```python
from build123d import *

# Parameters (mm, degrees)
BOSS_EXTRUDE1_DEPTH = 9
SHELL2_T            = -3
SKETCH3_W           = 14
SKETCH3_H           = 56
SKETCH3_W_2         = 12
SKETCH3_H_2         = 54
BOSS_EXTRUDE3_DEPTH = 6
FILLET1_R           = 5
FILLET5_R           = 5
FILLET8_R           = 0.5
FILLET9_R           = 3
FILLET10_R          = 2


with BuildPart() as part:
    # Sketch1 → Boss-Extrude1 (new, symmetric)
    with BuildSketch(Plane.YZ):
        with BuildLine():
            Line((0, 30), (-7.5, 30))
            ThreePointArc((-7.5, 30), (-15, 0), (-7.5, -30))
            Line((-7.5, -30), (0, -30))
            Line((0, -30), (0, 30))
        make_face()
    extrude(amount=BOSS_EXTRUDE1_DEPTH, both=True)

    # Shell2
    shell2_openings = [part.faces().sort_by_distance(p)[0] for p in [
        (0, 0, 0),
    ]]
    offset(amount=SHELL2_T, openings=shell2_openings, kind=Kind.INTERSECTION)

    # Sketch3 → Boss-Extrude3 (add, symmetric)
    with BuildSketch(Plane(origin=(0, 0, 0), x_dir=(-1, 0, 0), z_dir=(0, 1, 0))):
        Rectangle(SKETCH3_W, SKETCH3_H)
        Rectangle(SKETCH3_W_2, SKETCH3_H_2, mode=Mode.SUBTRACT)
    extrude(amount=BOSS_EXTRUDE3_DEPTH, both=True)

    # Fillet1
    fillet1_edges = [part.edges().sort_by_distance(p)[0] for p in [
        (0, -7.5, -30),
        (0, -7.5, 30),
    ]]
    fillet(fillet1_edges, radius=FILLET1_R)

    # Fillet5
    fillet5_edges = [part.edges().sort_by_distance(p)[0] for p in [
        (9, -2.207712898, 30),
        (-9, -2.207712898, -30),
        (9, -2.207712898, -30),
        (-9, -15, 0),
        (-9, -7.095136799, 29.221273379),
        (-9, -2.207712898, 30),
        (-9, -7.095136799, -29.221273379),
        (9, -15, 0),
        (9, -7.095136799, 29.221273379),
        (9, -7.095136799, -29.221273379),
    ]]
    fillet(fillet5_edges, radius=FILLET5_R)

    # Fillet8
    fillet8_edges = [part.edges().sort_by_distance(p)[0] for p in [
        (0, 0, 30),
        (-9, 0, 0),
        (9, 0, 0),
        (0, 0, -30),
        (7.535533906, 0, -28.535533906),
        (7.535533906, 0, 28.535533906),
        (-7.535533906, 0, -28.535533906),
        (-7.535533906, 0, 28.535533906),
    ]]
    fillet(fillet8_edges, radius=FILLET8_R)

    # Fillet9
    fillet9_edges = [part.edges().sort_by_distance(p)[0] for p in [
        (-7, 3, 28),
        (7, 3, 28),
        (7, 3, -28),
        (-7, 3, -28),
    ]]
    fillet(fillet9_edges, radius=FILLET9_R)

    # Fillet10
    fillet10_edges = [part.edges().sort_by_distance(p)[0] for p in [
        (-6, 0.164880099, 27),
        (-6, 0.164880099, -27),
        (6, 0.164880099, 27),
        (6, 0.164880099, -27),
    ]]
    fillet(fillet10_edges, radius=FILLET10_R)


solid = part.part
```
Input: part model. Units: mm. Frame: model coordinates. A direction names the side the tool comes from. Coordinates: 2 decimals unless noted, no trailing zeros. Write each loop counter-clockwise with the first axis right and the second up, starting at its lowest first coordinate (ties: lowest second). Pieces come first, ordered by that corner, then holes.
1) Material intervals for line 1 along Z through (x, y) = (-2.75, -4.75); line 2 along X through (y, z) = (-7.5, -16.5); line 3 along X through (y, z) = (1, -24), sorted ascending.
2) Section A-A on y = -1.5. Output: boundary loops of the cut face in (x, z).
3) Set-up query: faces 1 (the flat face through (7, 3, 0)), 2 (the flat face through (0, 3, -28)), 3 (the cylindrical face through (6.1, 2.96, 27.14)), 4 (the cylindrical face through (-6.1, 3.04, -27.14)), 5 (the cylindrical face through (0, -12, 0)). Return all of +Z, -Z, +X, -X, +Y, -Y with unobstructed straight access to the full face (end or side cutting, diameter ignored); none if empty.
4) Pin query (flat end, axial travel): pin 1 Ø6.5 at (x, y) = (1, 3) entering from +Z; pin 2 Ø3 at (y, z) = (2.5, 5.5) entering from +X; pin 3 Ø8 at (x, z) = (7, 14.5) entering from -Y. Return the tip coordinate at first contact, or that it passes through.
5) Mould query, pull axis Z, two halves, no side actions, for faces 6 (the flat face through (0, 0, -27)), 7 (the cylindrical face through (-6.14, 2.96, 27.1)), 8 (the flat face through (0, -2, -30)). Classes: pulls with the +Z half, pulls with the -Z half, needs draft (parallel to the pull), parting line crosses it, or undercut.
6) Section C-C on y = 2.5. Output: boundary loops of the cut face in (x, z).
7) Section B-B on x = -0.25. Output: boundary loops of the cut face in (y, z), and give its area (3 significant figures).
Check result:
1. line 1: z = -29.99 to -27, 27 to 29.99
1. line 2: x = -9 to -6, 6 to 9
1. line 3: x = -7 to -6, 6 to 7
2. outline: (-9, -25) arc R5 ccw to (-4, -30) - (4, -30) arc R5 ccw to (9, -25) - (9, 25) arc R5 ccw to (4, 30) - (-4, 30) arc R5 ccw to (-9, 25) - close; hole (-6, -25) arc R2 ccw to (-4, -27) - (4, -27) arc R2 ccw to (6, -25) - (6, 25) arc R2 ccw to (4, 27) - (-4, 27) arc R2 ccw to (-6, 25) - close
3. face 1: +Z, -Z, +X, +Y
3. face 2: -Z, +X, -X, +Y
3. face 3: +Z, +X, +Y
3. face 4: -Z, -X, +Y
3. face 5: +Y
4. pin 1: stops at z = 29.93
4. pin 2: stops at x = 7
4. pin 3: stops at y = -13.95
5. face 6: undercut
5. face 7: pulls with the +Z half
5. face 8: pulls with the -Z half
6. outline: (-7, -25) arc R3 ccw to (-4, -28) - (4, -28) arc R3 ccw to (7, -25) - (7, 25) arc R3 ccw to (4, 28) - (-4, 28) arc R3 ccw to (-7, 25) - close; hole (-6, -25) arc R2 ccw to (-4, -27) - (4, -27) arc R2 ccw to (6, -25) - (6, 25) arc R2 ccw to (4, 27) - (-4, 27) arc R2 ccw to (-6, 25) - close
7. outline: (-8.94, -27.13) arc R5 ccw to (-4.42, -30) - (-0.5, -30) arc R0.5 ccw to (0, -29.5) - (0, -28) - (6, -28) - (6, -27) - (-5.67, -27) arc R60.75 cw to (-5.67, 27) - (6, 27) - (6, 28) - (0, 28) - (0, 29.5) arc R0.5 ccw to (-0.5, 30) - (-4.42, 30) arc R5 ccw to (-8.94, 27.13) arc R63.75 ccw to start
7. area: 226 mm2
